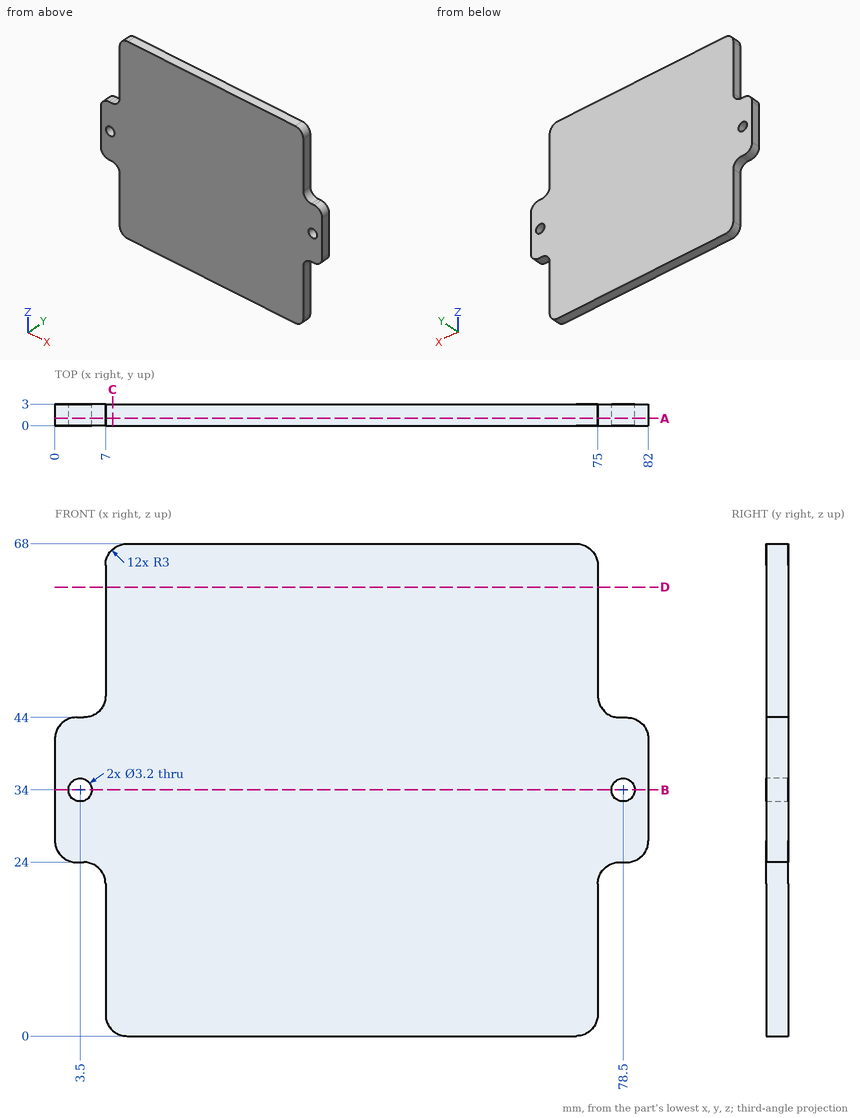
Study the drawing (mm; zero at the part's minimum x, y, z) and answer. Give positions to 0.01 mm unless a question says otherwise; leave off trailing zeros. Loops run counter-clockwise (first coordinate to the right, second up) from the corner with the lowest first, then second, coordinate; pieces in that order, holes last. Notation, with made-up numbers: (34, 37) - (49, 37) arc R14 cw to (49, 52) - close; hole circle Ø10 at (80.25, 5). An arc over 180 degrees is marked (long way). Answer in a Markdown table with one row per item. Add a question column.
Q1. The part is cut by section A-A (y = 1). Determine the outline of the cut face in (x, z).
Q2. The part is cut by section B-B (z = 34). Determine the outline of the cut face in (x, y).
Q3. The part is cut by section D-D (z = 62). Determine the outline of the cut face in (x, y), and give its area (3 significant figures).
Q4. Consider line 1 along X through (y, z) = (1.65, 34); line 2 along Z through (x, y) = (3.5, 1.9); line 3 along X through (y, z) = (0.3, 56.5). Determine where each line is inside the solid, lowest interval first.
Q5. The part is cut by section C-C (x = 8). Determine the outline of the cut face in (y, z).
Q6. Each of these flat-tipped pins is pushed along its axis until it touches: P1, Ø0.9, axis at y = 2, z = 8.5, coming from the +X side; P2, Ø2.5, axis at x = 3.5, z = 34, coming from the -Y side; P3, Ø0.8, axis at x = 3.5, y = 2, coming from the -Z side; P4, Ø0.9, axis at y = 1, z = 16, coming from the -X side. Where does it stop, or does it pass through?
Solution:
| question | item | result |
|---|---|---|
| 1 | outline | (0, 27) arc R3 ccw to (3, 24) - (4, 24) arc R3 cw to (7, 21) - (7, 3) arc R3 ccw to (10, 0) - (72, 0) arc R3 ccw to (75, 3) - (75, 21) arc R3 cw to (78, 24) - (79, 24) arc R3 ccw to (82, 27) - (82, 41) arc R3 ccw to (79, 44) - (78, 44) arc R3 cw to (75, 47) - (75, 65) arc R3 ccw to (72, 68) - (10, 68) arc R3 ccw to (7, 65) - (7, 47) arc R3 cw to (4, 44) - (3, 44) arc R3 ccw to (0, 41) - close; hole circle Ø3.2 at (3.5, 34); hole circle Ø3.2 at (78.5, 34) |
| 2 | outline | (0, 0) - (1.9, 0) - (1.9, 3) - (0, 3) - close; (5.1, 0) - (76.9, 0) - (76.9, 3) - (5.1, 3) - close; (80.1, 0) - (82, 0) - (82, 3) - (80.1, 3) - close |
| 3 | outline | (7, 0) - (75, 0) - (75, 3) - (7, 3) - close |
| 3 | area | 204 mm² |
| 4 | line 1 | x = 0 to 1.9, 5.1 to 76.9, 80.1 to 82 |
| 4 | line 2 | z = 24 to 32.4, 35.6 to 44 |
| 4 | line 3 | x = 7 to 75 |
| 5 | outline | (0, 0.76) - (3, 0.76) - (3, 67.24) - (0, 67.24) - close |
| 6 | P1 | stops at x = 75 |
| 6 | P2 | passes through |
| 6 | P3 | stops at z = 24 |
| 6 | P4 | stops at x = 7 |
